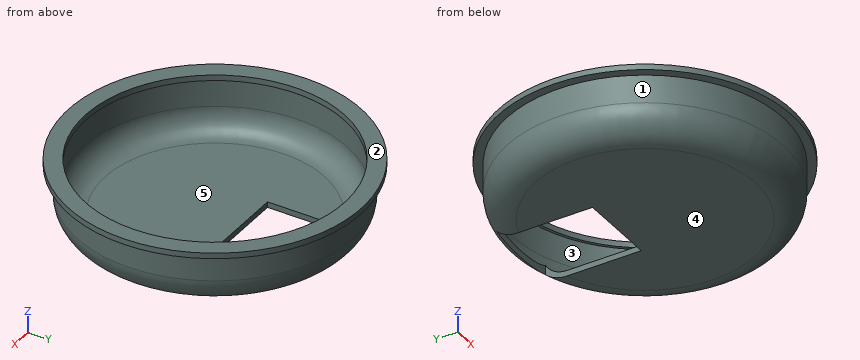
from build123d import *

# Parameters (mm, degrees)
BOX_W         = 14
BOX_H         = 17
BOX_DEPTH     = 6
SKETCH_R      = 24.5
PAD_DEPTH     = 10
FILLET_R      = 5
THICKNESS_T   = -1
SKETCH001_R   = 26
SKETCH001_R_2 = 23
PAD001_DEPTH  = 1


with BuildPart() as cube:
    # Box → Box (new body)
    with BuildSketch(Plane(origin=(-7, 5, -2), x_dir=(1, 0, 0), z_dir=(0, 0, 1))):
        with Locations((7, 8.5)):
            Rectangle(BOX_W, BOX_H)
    extrude(amount=BOX_DEPTH)


with BuildPart() as cut:
    # Sketch → Pad (new body)
    with BuildSketch(Plane.XY):
        Circle(SKETCH_R)
    extrude(amount=PAD_DEPTH)

    # Fillet
    fillet_edges = [cut.edges().sort_by_distance(p)[0] for p in [
        (-24.5, 0, 0),
    ]]
    fillet(fillet_edges, radius=FILLET_R)

    # Thickness
    thickness_openings = [cut.faces().sort_by_distance(p)[0] for p in [
        (0, 0, 10),
    ]]
    offset(amount=THICKNESS_T, openings=thickness_openings)

    # Sketch001 → Pad001 (new body)
    with BuildSketch(Plane.XY.offset(10)):
        Circle(SKETCH001_R)
        Circle(SKETCH001_R_2, mode=Mode.SUBTRACT)
    extrude(amount=PAD001_DEPTH)

    # Cut: cut Cube
    add(cube.part, mode=Mode.SUBTRACT)


solid = cut.part
Work out the finished part from the listing and answer in its coordinate system (mm). Face numbers are marked on the shaded views. A direction names the side the tool comes from. Give positions to 0.01 mm unless a question says otherwise; leave off trailing zeros. Loops run counter-clockwise (first coordinate to the right, second up) from the corner with the lowest first, then second, coordinate; pieces in that order, holes last. Notation, with made-up numbers: (50, -39) - (81, -39) arc R25 ccw to (81, -2) - close; hole circle Ø7 at (40.25, 47). An arc over 180 degrees is marked (long way). Answer in a Markdown table with one row per item. Add a question column.
Q1. Each of these flat-tipped pins is pushed along its axis until it touches: P1, Ø1.5, axis at y = -15, z = 9, coming from the -X side; P2, Ø6, axis at x = -3.5, y = 0.5, coming from the +Z side; P3, Ø10, axis at x = -10.5, y = -2, coming from the -Z side; P4, Ø4, axis at y = 12, z = 7, coming from the -X side. Where does it stop, or does it pass through?
Q2. The part is cut by section A-A (y = 0). Determine the outline of the cut face in (x, z).
Q3. The part is cut by section C-C (z = 2.5). Determine the outline of the cut face in (x, y) (1 decimal), and give its area (3 significant figures).
Q4. Determine the mould class of the marked faces 1, 2 and 3 for opening direction Y: released by +Y, released by -Y, zero draft, split by the parting line, or undercut.
Q5. Consider line 1 along Y through (x, z) = (0, 8.8); line 2 along Y through (x, z) = (0, 10.2); line 3 along Z through (x, y) = (14, -13). Determine where each line is inside the solid, lowest interval first.
Q6. A tool of negligible diameter and unlimited length cuts with its end or side. For the marked faces 4 and 5, from which of +Z, -Z, +X, -X, +Y, -Y can it reach the whole face along a straight path? Write none if from no direction.
Q7. The part is cut by section D-D (z = 6.5). Determine the outline of the cut face in (x, y), and give its area (3 significant figures).
Q8. The part is cut by section B-B (x = 0). Determine the outline of the cut face in (y, z).
Solution:
| question | item | result |
|---|---|---|
| 1 | P1 | stops at x = -19.93 |
| 1 | P2 | stops at z = 1 |
| 1 | P3 | stops at z = 0 |
| 1 | P4 | stops at x = -22.37 |
| 2 | outline | (-26, 10) - (-24.5, 10) - (-24.5, 5) arc R5 ccw to (-19.5, 0) - (19.5, 0) arc R5 ccw to (24.5, 5) - (24.5, 10) - (26, 10) - (26, 11) - (23, 11) - (23, 10) - (23.5, 10) - (23.5, 5) arc R4 cw to (19.5, 1) - (-19.5, 1) arc R4 cw to (-23.5, 5) - (-23.5, 10) - (-23, 10) - (-23, 11) - (-26, 11) - close |
| 3 | outline | circle Ø47.7 at (0, 0); hole (-7, 21.5) arc R22.6 ccw (long way) to (7, 21.5) - (7, 22) - (5.3, 22) arc R22.6 ccw to (-5.3, 22) - (-7, 22) - close |
| 3 | area | 175 mm² |
| 4 | face 1 | split by the parting line |
| 4 | face 2 | zero draft |
| 4 | face 3 | undercut |
| 5 | line 1 | y = -24.5 to -23.5, 23.5 to 24.5 |
| 5 | line 2 | y = -26 to -23, 23 to 26 |
| 5 | line 3 | z = 0 to 1 |
| 6 | face 4 | -Z, +X, -X, +Y, -Y |
| 6 | face 5 | +Z |
| 7 | outline | circle Ø49 at (0, 0); hole circle Ø47 at (0, 0) |
| 7 | area | 151 mm² |
| 8 | outline | (-26, 10) - (-24.5, 10) - (-24.5, 5) arc R5 ccw to (-19.5, 0) - (5, 0) - (5, 1) - (-19.5, 1) arc R4 cw to (-23.5, 5) - (-23.5, 10) - (-23, 10) - (-23, 11) - (-26, 11) - close; (22, 0.67) arc R5 ccw to (24.5, 5) - (24.5, 10) - (26, 10) - (26, 11) - (23, 11) - (23, 10) - (23.5, 10) - (23.5, 5) arc R4 cw to (22, 1.88) - close |
